from build123d import *

# Parameters (mm, degrees)
SKETCH1_R           = 10.679205769
BOSS_EXTRUDE1_DEPTH = 7
CUT_EXTRUDE1_START  = -5
SKETCH2_R           = 10.679205769
SKETCH2_R_2         = 10
CUT_EXTRUDE1_DEPTH  = 5


with BuildPart() as part:
    # Sketch1 → Boss-Extrude1 (new body)
    with BuildSketch(Plane.XY):
        Circle(SKETCH1_R)
        with BuildLine():
            Line((-1.732050808, 1), (1.732050808, 1))
            ThreePointArc((1.732050808, 1), (0, -2), (-1.732050808, 1))
        make_face(mode=Mode.SUBTRACT)
    extrude(amount=BOSS_EXTRUDE1_DEPTH)

    # Sketch2 → Cut-Extrude1 (cut)
    with BuildSketch(Plane.XY.offset(6).offset(CUT_EXTRUDE1_START)):
        Circle(SKETCH2_R)
        Circle(SKETCH2_R_2, mode=Mode.SUBTRACT)
    extrude(amount=CUT_EXTRUDE1_DEPTH, mode=Mode.SUBTRACT)


solid = part.part
Geometry check sheet. Reference: the model listing, model coordinates, mm. A direction names the side the tool comes from. Give positions to 0.01 mm unless a question says otherwise; leave off trailing zeros. Order: outer loops, then holes, each group sorted by start corner. A loop starts at its lowest first (then second) coordinate and runs counter-clockwise, first axis right, second up.
1) Draft check along Z on faces 1 (the cylindrical face through (0, -2, 3)), 2 (the cylindrical face through (-2.17, -9.76, 3.46)), 3 (the flat face through (-0.1, -2.2, 7)). Enter one of: released by +Z, released by -Z, zero draft, split by the parting line, or undercut.
Results are:
face 1: zero draft
face 2: undercut
face 3: released by +Z
2) Gauge pin test, flat ends, axial feed: pin 1 (3 mm diameter, centred on y = -4, z = 1, fed in from +X); pin 2 (4.5 mm diameter, centred on x = 0, y = 0, fed in from +Z); pin 3 (1 mm diameter, centred on y = 1, z = 4.5, fed in from +X); pin 4 (1.7 mm diameter, centred on x = -0.5, z = 4, fed in from -Y). Record the tip position at first contact, or that the pin passes through.
Results are:
pin 1: stops at x = 10.38
pin 2: stops at z = 7
pin 3: stops at x = 9.99
pin 4: stops at y = -10
3) Tool access check on faces 4 (the flat face through (0, 1, 3)), 5 (the flat face through (3, 10, 1)), 6 (the flat face through (-0.1, -2.2, 0)). Record the directions out of +Z, -Z, +X, -X, +Y, -Y that give a thin tool (end or side, any length) a straight path to the whole face; none if there is none.
Results are:
face 4: +Z, -Z
face 5: none
face 6: -Z, +X, -X, +Y, -Y
4) Material ranges on probe 1 along Y at (x, z) = (-0.75, 4.5); probe 2 along X at (y, z) = (-1.5, 4.25); probe 3 along Y at (x, z) = (-0.75, 6.75), recorded low to high.
Results are:
probe 1: y = -9.97 to -1.85, 1 to 9.97
probe 2: x = -9.89 to -1.32, 1.32 to 9.89
probe 3: y = -10.65 to -1.85, 1 to 10.65
5) Cross-section at B-B (x = 0.5). Record the boundary of the cut face in (y, z), then the cut area to 3 significant figures.
Results are:
outline: (-10.67, 0) - (-1.94, 0) - (-1.94, 7) - (-10.67, 7) - (-10.67, 6) - (-9.99, 6) - (-9.99, 1) - (-10.67, 1) - close; (1, 0) - (10.67, 0) - (10.67, 1) - (9.99, 1) - (9.99, 6) - (10.67, 6) - (10.67, 7) - (1, 7) - close
area: 122 mm2
6) Cross-section at D-D (x = -2.25). Record the boundary of the cut face in (y, z), then the cut area to 3 significant figures.
Results are:
outline: (-10.44, 0) - (10.44, 0) - (10.44, 1) - (9.74, 1) - (9.74, 6) - (10.44, 6) - (10.44, 7) - (-10.44, 7) - (-10.44, 6) - (-9.74, 6) - (-9.74, 1) - (-10.44, 1) - close
area: 139 mm2
7) Cross-section at C-C (z = 1.75). Record the boundary of the cut face in (x, y), then the cut area to 3 significant figures.
Results are:
outline: circle Ø20 at (0, 0); hole (-1.73, 1) arc R2 ccw (long way) to (1.73, 1) - close
area: 304 mm2
8) Cross-section at A-A (y = 0). Record the boundary of the cut face in (x, z).
Results are:
outline: (-10.68, 0) - (-2, 0) - (-2, 7) - (-10.68, 7) - (-10.68, 6) - (-10, 6) - (-10, 1) - (-10.68, 1) - close; (2, 0) - (10.68, 0) - (10.68, 1) - (10, 1) - (10, 6) - (10.68, 6) - (10.68, 7) - (2, 7) - close
